Can you work these out from the drawing? Everything is in mm from the part's minimum corner. Round coordinates to 2 decimals unless told otherwise and drop trailing zeros. Write each loop counter-clockwise with the first axis right and the second up, starting at its lowest first coordinate (ties: lowest second). Pieces come first, ordered by that corner, then holes. Notation, with made-up numbers: (33, -12.5) - (76, -12.5) arc R14 ccw to (76, 13.5) - close; hole circle Ø7 at (16, 29.5). An arc over 180 degrees is marked (long way). One line per item, written item: value. Start each with the question number.
(1) I want a section at C-C on z = 10.75. List the corners of the cut face in (x, y) for me.
(2) If I drill on L1, parallel to Z at x = 9, y = 2.6; L2, parallel to X at y = 0.7, z = 10.5; L3, parallel to X at y = 2.65, z = 10.25, over which ranges is the centre line in solid material (lowest first)? Write a range as from..to.
(3) I want a section at A-A on x = 7.5. List the corners of the cut face in (y, z) for me.
(4) I'm going to push a flat-ended pin straight in: pin 1 Ø1.5 at (y, z) = (2.5, 6.5) entering from +X. Where does the tip first touch, or does it pass through?
(5) Thinking about a two-plate mould opening in X: for the marked faces 1, 2 and 3, which applies, +X half, -X half, draft (parallel to the pull), parting line (faces both ways), or undercut?
(6) I want a section at D-D on z = 13. List the corners of the cut face in (x, y) for me, plus the area to 3 significant figures.
(7) I want a section at B-B on y = 5.5. List the corners of the cut face in (x, z) for me.
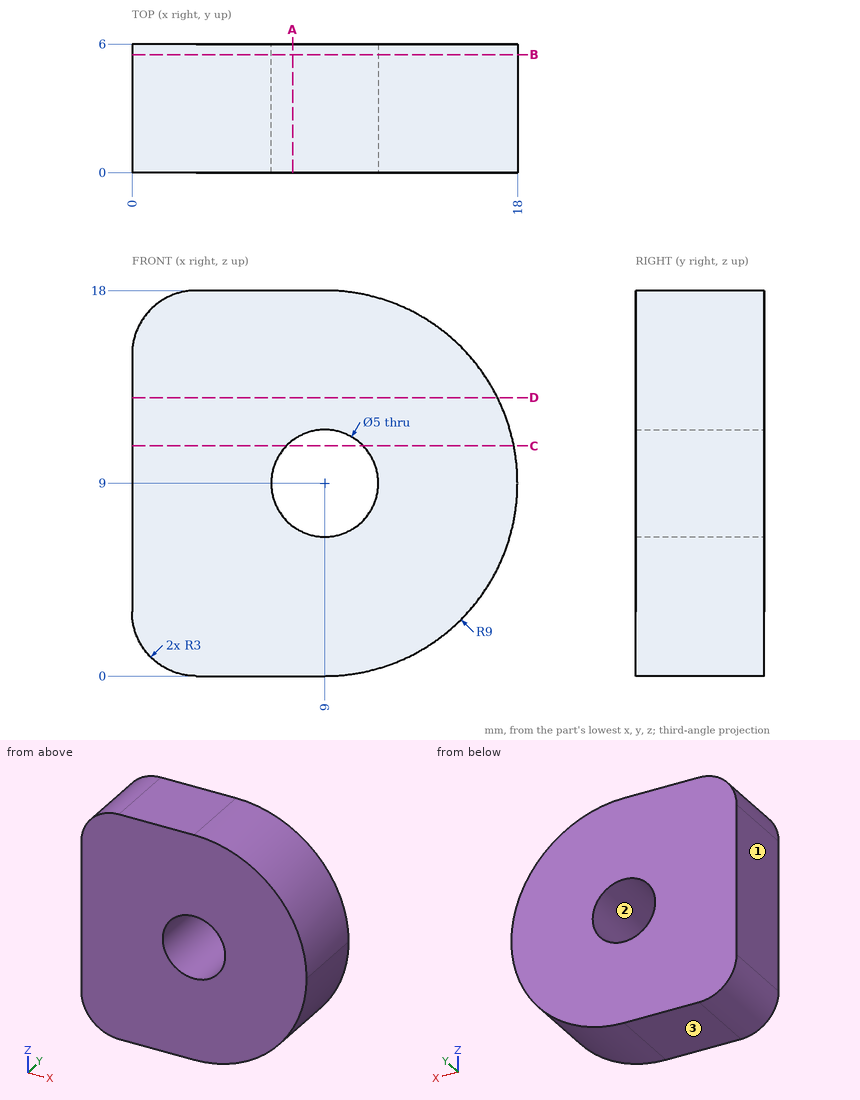
Established:
1. outline: (0, 0) - (7.21, 0) - (7.21, 6) - (0, 6) - close; (10.79, 0) - (17.83, 0) - (17.83, 6) - (10.79, 6) - close
2. L1: 0..6.5, 11.5..18
2. L2: 0..7, 11..17.87
2. L3: 0..6.83, 11.17..17.91
3. outline: (0, 0) - (6, 0) - (6, 7) - (0, 7) - close; (0, 11) - (6, 11) - (6, 18) - (0, 18) - close
4. pin 1: x = 17.83
5. face 1: -X half
5. face 2: undercut
5. face 3: draft
6. outline: (0, 0) - (17.06, 0) - (17.06, 6) - (0, 6) - close
6. area: 102 mm2
7. outline: (0, 3) arc R3 ccw to (3, 0) - (9, 0) arc R9 ccw to (9, 18) - (3, 18) arc R3 ccw to (0, 15) - close; hole circle Ø5 at (9, 9)
